Work out the finished part from the listing and answer in its coordinate system (mm). Face numbers are marked on the shaded views. A direction names the side the tool comes from. Coordinates: 2 decimals unless noted, no trailing zeros. Order: outer loops, then holes, each group sorted by start corner. A loop starts at its lowest first (then second) coordinate and runs counter-clockwise, first axis right, second up. Notation, with made-up numbers: M -19.75,-11 L 36.25,-11 A21 cw 36.25,19 Z; hole C 66.25,-12 d11. An arc over 180 degrees is marked long. Use a Markdown table: item, result.
Autodesk Inventor part; units mm, degrees
ref_plane "YZ Plane" through (0, 0, 0) normal (1, 0, 0) x (0, 1, 0)
ref_plane "XZ Plane" through (0, 0, 0) normal (0, 1, 0) x (-1, 0, 0)
ref_plane "XY Plane" through (0, 0, 0) normal (0, 0, 1) x (1, 0, 0)
sketch "Sketch1" plane through (0, 0, 0) normal (1, 0, 0) x (0, 1, 0)
  circle A0 centre (2.2464, -2.4677) radius 12.5
  circle A1 centre (2.2464, -2.4677) radius 2
  arc A2 (9.603, -3.2677) -> (9.603, -1.6677) centre (2.2464, -2.4677) ccw
  arc A3 (12.9165, -3.2677) -> (12.9165, -1.6677) centre (2.2464, -2.4677) ccw
  line L0 (9.603, -3.2677) -> (12.9165, -3.2677)
  line L1 (9.603, -1.6677) -> (12.9165, -1.6677)
  line L2 (8.9958, 0.5665) -> (12.147, 1.5904)
  arc A4 (12.6414, 0.0687) -> (12.147, 1.5904) centre (2.2464, -2.4677) ccw
  line L3 (9.4902, -0.9552) -> (12.6414, 0.0687)
  arc A5 (9.4902, -0.9552) -> (8.9958, 0.5665) centre (2.2464, -2.4677) ccw
  line L4 (7.7278, 2.5037) -> (10.4084, 4.4513)
  arc A6 (11.3489, 3.1568) -> (10.4084, 4.4513) centre (2.2464, -2.4677) ccw
  line L5 (8.6683, 1.2092) -> (11.3489, 3.1568)
  arc A7 (8.6683, 1.2092) -> (7.7278, 2.5037) centre (2.2464, -2.4677) ccw
  line L6 (5.9233, 3.9542) -> (7.8709, 6.6348)
  arc A8 (9.1653, 5.6944) -> (7.8709, 6.6348) centre (2.2464, -2.4677) ccw
  line L7 (7.2177, 3.0138) -> (9.1653, 5.6944)
  arc A9 (7.2177, 3.0138) -> (5.9233, 3.9542) centre (2.2464, -2.4677) ccw
  line L8 (3.7589, 4.7761) -> (4.7828, 7.9274)
  arc A10 (6.3045, 7.433) -> (4.7828, 7.9274) centre (2.2464, -2.4677) ccw
  line L9 (5.2806, 4.2817) -> (6.3045, 7.433)
  arc A11 (5.2806, 4.2817) -> (3.7589, 4.7761) centre (2.2464, -2.4677) ccw
  line L10 (1.4464, 4.889) -> (1.4464, 8.2024)
  arc A12 (3.0464, 8.2024) -> (1.4464, 8.2024) centre (2.2464, -2.4677) ccw
  line L11 (3.0464, 4.889) -> (3.0464, 8.2024)
  arc A13 (3.0464, 4.889) -> (1.4464, 4.889) centre (2.2464, -2.4677) ccw
  line L12 (-0.7878, 4.2817) -> (-1.8117, 7.433)
  arc A14 (-0.29, 7.9274) -> (-1.8117, 7.433) centre (2.2464, -2.4677) ccw
  line L13 (0.7339, 4.7761) -> (-0.29, 7.9274)
  arc A15 (0.7339, 4.7761) -> (-0.7878, 4.2817) centre (2.2464, -2.4677) ccw
  line L14 (-2.7249, 3.0138) -> (-4.6725, 5.6944)
  arc A16 (-3.3781, 6.6348) -> (-4.6725, 5.6944) centre (2.2464, -2.4677) ccw
  line L15 (-1.4305, 3.9542) -> (-3.3781, 6.6348)
  arc A17 (-1.4305, 3.9542) -> (-2.7249, 3.0138) centre (2.2464, -2.4677) ccw
  line L16 (-4.1755, 1.2092) -> (-6.8561, 3.1568)
  arc A18 (-5.9156, 4.4513) -> (-6.8561, 3.1568) centre (2.2464, -2.4677) ccw
  line L17 (-3.235, 2.5037) -> (-5.9156, 4.4513)
  arc A19 (-3.235, 2.5037) -> (-4.1755, 1.2092) centre (2.2464, -2.4677) ccw
  line L18 (-4.9974, -0.9552) -> (-8.1486, 0.0687)
  arc A20 (-7.6542, 1.5904) -> (-8.1486, 0.0687) centre (2.2464, -2.4677) ccw
  line L19 (-4.503, 0.5665) -> (-7.6542, 1.5904)
  arc A21 (-4.503, 0.5665) -> (-4.9974, -0.9552) centre (2.2464, -2.4677) ccw
  line L20 (-5.1102, -3.2677) -> (-8.4237, -3.2677)
  arc A22 (-8.4237, -1.6677) -> (-8.4237, -3.2677) centre (2.2464, -2.4677) ccw
  line L21 (-5.1102, -1.6677) -> (-8.4237, -1.6677)
  arc A23 (-5.1102, -1.6677) -> (-5.1102, -3.2677) centre (2.2464, -2.4677) ccw
  line L22 (-4.503, -5.5018) -> (-7.6542, -6.5257)
  arc A24 (-8.1486, -5.004) -> (-7.6542, -6.5257) centre (2.2464, -2.4677) ccw
  line L23 (-4.9974, -3.9801) -> (-8.1486, -5.004)
  arc A25 (-4.9974, -3.9801) -> (-4.503, -5.5018) centre (2.2464, -2.4677) ccw
  line L24 (-3.235, -7.439) -> (-5.9156, -9.3866)
  arc A26 (-6.8561, -8.0921) -> (-5.9156, -9.3866) centre (2.2464, -2.4677) ccw
  line L25 (-4.1755, -6.1446) -> (-6.8561, -8.0921)
  arc A27 (-4.1755, -6.1446) -> (-3.235, -7.439) centre (2.2464, -2.4677) ccw
  line L26 (-1.4305, -8.8895) -> (-3.3781, -11.5701)
  arc A28 (-4.6725, -10.6297) -> (-3.3781, -11.5701) centre (2.2464, -2.4677) ccw
  line L27 (-2.7249, -7.9491) -> (-4.6725, -10.6297)
  arc A29 (-2.7249, -7.9491) -> (-1.4305, -8.8895) centre (2.2464, -2.4677) ccw
  line L28 (0.7339, -9.7114) -> (-0.29, -12.8627)
  arc A30 (-1.8117, -12.3683) -> (-0.29, -12.8627) centre (2.2464, -2.4677) ccw
  line L29 (-0.7878, -9.217) -> (-1.8117, -12.3683)
  arc A31 (-0.7878, -9.217) -> (0.7339, -9.7114) centre (2.2464, -2.4677) ccw
  line L30 (3.0464, -9.8243) -> (3.0464, -13.1377)
  arc A32 (1.4464, -13.1377) -> (3.0464, -13.1377) centre (2.2464, -2.4677) ccw
  line L31 (1.4464, -9.8243) -> (1.4464, -13.1377)
  arc A33 (1.4464, -9.8243) -> (3.0464, -9.8243) centre (2.2464, -2.4677) ccw
  line L32 (5.2806, -9.217) -> (6.3045, -12.3683)
  arc A34 (4.7828, -12.8627) -> (6.3045, -12.3683) centre (2.2464, -2.4677) ccw
  line L33 (3.7589, -9.7114) -> (4.7828, -12.8627)
  arc A35 (3.7589, -9.7114) -> (5.2806, -9.217) centre (2.2464, -2.4677) ccw
  line L34 (7.2177, -7.9491) -> (9.1653, -10.6297)
  arc A36 (7.8709, -11.5701) -> (9.1653, -10.6297) centre (2.2464, -2.4677) ccw
  line L35 (5.9233, -8.8895) -> (7.8709, -11.5701)
  arc A37 (5.9233, -8.8895) -> (7.2177, -7.9491) centre (2.2464, -2.4677) ccw
  line L36 (8.6683, -6.1446) -> (11.3489, -8.0921)
  arc A38 (10.4084, -9.3866) -> (11.3489, -8.0921) centre (2.2464, -2.4677) ccw
  line L37 (7.7278, -7.439) -> (10.4084, -9.3866)
  arc A39 (7.7278, -7.439) -> (8.6683, -6.1446) centre (2.2464, -2.4677) ccw
  line L38 (9.4902, -3.9801) -> (12.6414, -5.004)
  arc A40 (12.147, -6.5257) -> (12.6414, -5.004) centre (2.2464, -2.4677) ccw
  line L39 (8.9958, -5.5018) -> (12.147, -6.5257)
  arc A41 (8.9958, -5.5018) -> (9.4902, -3.9801) centre (2.2464, -2.4677) ccw
  point P0 (0, 0)
  dimension "d7" = 5.4
  dimension "d12" = 360
extrude "Extrusion1" add sketch "Sketch1" along normal blind 3
properties part number "Enc_"
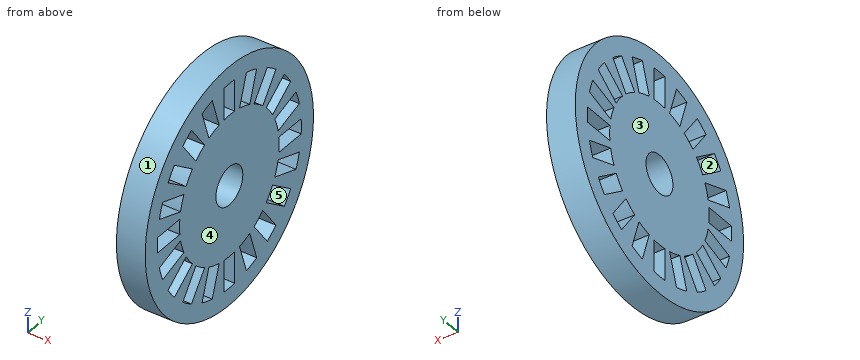
(1) Which of the six approach directions +Z, -Z, +X, -X, +Y, -Y give full straight-line access (tool end or side, diameter ignored) to the marked faces 4 and 5?
Conclusion:
| item | result |
|---|---|
| face 4 | +Z, -Z, +X, +Y, -Y |
| face 5 | +X, -X |
(2) Determine the mould class of the marked faces 1, 2 and 3 for opening direction Z: pulls with the +Z half, pulls with the -Z half, needs draft (parallel to the pull), parting line crosses it, or undercut.
Conclusion:
| item | result |
|---|---|
| face 1 | parting line crosses it |
| face 2 | undercut |
| face 3 | needs draft |
(3) A cutting plane is placed at C-C (y = 8.25). Determine the outline of the cut face in (x, z), then the cut area to 3 significant figures.
Conclusion:
| item | result |
|---|---|
| outline | M 0,-13.43 L 3,-13.43 L 3,-11.32 L 0,-11.32 Z; M 0,-9.37 L 3,-9.37 L 3,-7.82 L 0,-7.82 Z; M 0,-6.79 L 3,-6.79 L 3,1.86 L 0,1.86 Z; M 0,2.88 L 3,2.88 L 3,4.43 L 0,4.43 Z; M 0,6.39 L 3,6.39 L 3,8.5 L 0,8.5 Z |
| area | 47.9 mm2 |
(4) Straight lines are drawn through the part: L1, parallel to Y at x = 1.6, z = -7.25; L2, parallel to Z at x = 1.2, y = -5.25 (3 decimals); L3, parallel to Y at x = 1.3, z = -7. For each, find the intervals that lie inside material, in ascending order.
Conclusion:
| item | result |
|---|---|
| L1 | -9.3 to -5.7, -3.4 to 7.89, 10.19 to 13.8 |
| L2 | -12.47 to -8.903, -6.925 to -5.745, -4.062 to -3.268, -1.668 to -0.873, 0.809 to 1.99, 3.968 to 7.535 |
| L3 | -9.4 to -5.35, -3.6 to 8.1, 9.85 to 13.9 |
(5) A cutting plane is placed at A-A (z = 6). Determine the outline of the cut face in (x, y), then the cut area to 3 significant figures.
Conclusion:
| item | result |
|---|---|
| outline | M 0,-6.95 L 3,-6.95 L 3,-4.29 L 0,-4.29 Z; M 0,-2.92 L 3,-2.92 L 3,-1.35 L 0,-1.35 Z; M 0,0.34 L 3,0.34 L 3,1.45 L 0,1.45 Z; M 0,3.05 L 3,3.05 L 3,4.16 L 0,4.16 Z; M 0,5.84 L 3,5.84 L 3,7.41 L 0,7.41 Z; M 0,8.79 L 3,8.79 L 3,11.44 L 0,11.44 Z |
| area | 32.0 mm2 |
(6) Given P1, Ø0.9, axis at x = 2, z = -11.5, coming from the -Y side; P2, Ø0.9, axis at x = 1.5, y = -7, coming from the -Z side; P3, Ø1.5, axis at x = 1.5, z = -11.5, coming from the +Y side, each flat-ended and moving along its own axis, determine where each tip first touches the part or whether it passes through.
Conclusion:
| item | result |
|---|---|
| P1 | y = -6.84 |
| P2 | z = -11.35 |
| P3 | y = 11.61 |
(7) A cutting plane is placed at B-B (y = 2). Determine the outline of the cut face in (x, z), then the cut area to 3 significant figures.
Conclusion:
| item | result |
|---|---|
| outline | M 0,-14.97 L 3,-14.97 L 3,-13.16 L 0,-13.16 Z; M 0,-9.86 L 3,-9.86 L 3,-4.45 L 0,-4.45 Z; M 0,-0.48 L 3,-0.48 L 3,4.93 L 0,4.93 Z; M 0,8.23 L 3,8.23 L 3,10.03 L 0,10.03 Z |
| area | 43.3 mm2 |
(8) A cutting plane is placed at D-D (y = -6.25). Determine the outline of the cut face in (x, z).
Conclusion:
| item | result |
|---|---|
| outline | M 0,-11.64 L 3,-11.64 L 3,-8.97 L 0,-8.97 Z; M 0,-7.65 L 3,-7.65 L 3,-6.07 L 0,-6.07 Z; M 0,-4.39 L 3,-4.39 L 3,-3.27 L 0,-3.27 Z; M 0,-1.67 L 3,-1.67 L 3,-0.55 L 0,-0.55 Z; M 0,1.13 L 3,1.13 L 3,2.72 L 0,2.72 Z; M 0,4.04 L 3,4.04 L 3,6.7 L 0,6.7 Z |
